```python
from build123d import *

# Parameters (mm, degrees)
PAD_DEPTH    = 50
SKETCH002_W  = 36.843056
SKETCH002_H  = 26
PAD003_DEPTH = 17.5
FILLET_R     = 2


with BuildPart() as pad:
    # Sketch → Pad (new body, symmetric)
    with BuildSketch(Plane.XZ):
        with BuildLine():
            Line((-13.5, 0), (13.5, 0))
            ThreePointArc((17.5, 0), (15.5, 2), (13.5, 0))
            ThreePointArc((-17.5, 0), (0, -17.5), (17.5, 0))
            ThreePointArc((-13.5, 0), (-15.5, 2), (-17.5, 0))
        make_face()
    extrude(amount=PAD_DEPTH, both=True)


with BuildPart() as fillet_body:
    # Sketch002 → Pad003 (new body, symmetric)
    with BuildSketch(Plane.XZ):
        with Locations((5.578472, -8)):
            Rectangle(SKETCH002_W, SKETCH002_H)
    extrude(amount=PAD003_DEPTH, both=True)

    # Cut: cut Pad
    add(pad.part, mode=Mode.SUBTRACT)

    # Fillet
    fillet_edges = [fillet_body.edges().sort_by_distance(p)[0] for p in [
        (-12.843056, 0, -11.887216),
    ]]
    fillet(fillet_edges, radius=FILLET_R)


solid = fillet_body.part
```
Part model, mm, in its own coordinate system. A direction names the side the tool comes from. Coordinates: 2 decimals unless noted, no trailing zeros. Order: outer loops, then holes, each group sorted by start corner. A loop starts at its lowest first (then second) coordinate and runs counter-clockwise, first axis right, second up. Notation, with made-up numbers: (-35, -4) - (3, -4) arc R23 cw to (3, 16) - close; hole circle Ø11 at (-14.5, 88). An arc over 180 degrees is marked (long way). Return JSON: item names as keys, results as strings. Group by question number.
Item 1: Cut at A-A (x = 0). List the corners of the cut face in (y, z), plus the area to 4 significant figures.
Item 2: Cut at D-D (z = -2). List the corners of the cut face in (x, y).
Item 3: Cut at C-C (y = 0.5). List the corners of the cut face in (x, z), plus the area to 3 significant figures.
Item 4: Cut at B-B (x = 7). List the corners of the cut face in (y, z), plus the area to 3 significant figures.
Item 5: Which spindle directions (+Z, -Z, +X, -X, +Y, -Y) get a long thin tool onto all of the face, cutting with end or side? Do faces 5 (the face through (24, 0, -8)), 6 (the face through (0, 0, 0)), 7 (the face through (-11.812, -0.245, -14.458)). Say none if no direction does.
Item 6: Drill centre lines: probe 1 along Z at (x, y) = (-11, -12); probe 2 along Z at (x, y) = (8, -9); probe 3 along X at (y, z) = (4.5, -15.25). Where is each one in solid material? Low to high. Write a range as from..to.
Item 7: Pull direction Z, two halves, no side cores. Call faces 1 (the face through (14, -17.5, -14)), 2 (the face through (5, 0, 5)), 3 (the face through (5, 0, -21)), 4 (the face through (15.5, -0.2, 2)): pulls with the +Z half, pulls with the -Z half, needs draft (parallel to the pull), parting line crosses it, or undercut.
Item 8: Pin check, flat tips, straight feed: pin 1 (1.5 mm diameter, centred on y = 10.5, z = -6.5, fed in from -X); pin 2 (3 mm diameter, centred on y = 1.5, z = -12, fed in from -X). Stop position of each tip, or through.
Check values:
{
 "1": {"outline": "(-17.5, -21) - (17.5, -21) - (17.5, -17.5) - (-17.5, -17.5) - close; (-17.5, 0) - (17.5, 0) - (17.5, 5) - (-17.5, 5) - close", "area": "297.5 mm2"},
 "2": {"outline": "(17.39, -17.5) - (24, -17.5) - (24, 17.5) - (17.39, 17.5) - close"},
 "3": {"outline": "(-12.84, -21) - (24, -21) - (24, 5) - (-12.84, 5) - (-12.84, 0) - (13.5, 0) arc R2 cw to (17.5, 0) arc R17.5 cw to (-9.73, -14.55) arc R2 ccw to (-12.84, -16.21) - close", "area": "505 mm2"},
 "4": {"outline": "(-17.5, -21) - (17.5, -21) - (17.5, -16.04) - (-17.5, -16.04) - close; (-17.5, 0) - (17.5, 0) - (17.5, 5) - (-17.5, 5) - close", "area": "349 mm2"},
 "5": {"face 5": "+Z, -Z, +X, +Y, -Y", "face 6": "-X, +Y, -Y", "face 7": "+Y, -Y"},
 "6": {"probe 1": "z = -21..-14.21, 0..5", "probe 2": "z = -21..-15.56, 0..5", "probe 3": "x = -12.6..-8.58, 8.58..24"},
 "7": {"face 1": "needs draft", "face 2": "pulls with the +Z half", "face 3": "pulls with the -Z half", "face 4": "undercut"},
 "8": {"pin 1": "stops at x = 15.93", "pin 2": "stops at x = 11.14"}
}
